Design review of the part built by this model. Coordinates are the model's own, in mm. A direction names the side the tool comes from. Coordinates: 2 decimals unless noted, no trailing zeros. Loops run counter-clockwise (first coordinate to the right, second up) from the corner with the lowest first, then second, coordinate; pieces in that order, holes last.
from build123d import *

# Parameters (mm, degrees)
F0_R     = 0.8
F1_DEPTH = 3
F2_R     = 0.8
F3_DEPTH = 30.501
F4_R     = 1


with BuildPart() as f1:
    # F0 (on Top) → F1 (new body)
    with BuildSketch(Plane.XY):
        with BuildLine():
            Line((13.5, 15.25), (-13.5, 15.25))
            ThreePointArc((-13.5, 15.25), (-14.56066, 14.81066), (-15, 13.75))
            Line((-15, 13.75), (-15, -13.75))
            ThreePointArc((-15, -13.75), (-14.56066, -14.81066), (-13.5, -15.25))
            Line((-13.5, -15.25), (13.5, -15.25))
            ThreePointArc((13.5, -15.25), (14.56066, -14.81066), (15, -13.75))
            Line((15, -13.75), (15, 13.75))
            ThreePointArc((15, 13.75), (14.56066, 14.81066), (13.5, 15.25))
        make_face()
        with Locations((-10, -10)):
            Circle(F0_R, mode=Mode.SUBTRACT)
        with Locations((10, -10)):
            Circle(F0_R, mode=Mode.SUBTRACT)
        with Locations((-10, 10)):
            Circle(F0_R, mode=Mode.SUBTRACT)
        with BuildLine():
            ThreePointArc((1.25, 9.921567), (7.5, 6.614378), (10, 0))
            ThreePointArc((10, 0), (7.5, -6.614378), (1.25, -9.921567))
            Line((1.25, -9.921567), (1.25, -10))
            ThreePointArc((1.25, -10), (0, -11.25), (-1.25, -10))
            Line((-1.25, -10), (-1.25, -9.921567))
            ThreePointArc((-1.25, -9.921567), (-10, 0), (-1.25, 9.921567))
            Line((-1.25, 9.921567), (-1.25, 10))
            ThreePointArc((-1.25, 10), (0, 11.25), (1.25, 10))
            Line((1.25, 10), (1.25, 9.921567))
        make_face(mode=Mode.SUBTRACT)
        with Locations((10, 10)):
            Circle(F0_R, mode=Mode.SUBTRACT)
    extrude(amount=F1_DEPTH)

    # F2 (on face) → F3 (cut, through all)
    with BuildSketch(Plane.XZ.offset(15.25)):
        with Locations((0, 1.5)):
            Circle(F2_R)
        with Locations((10, 1.5)):
            Circle(F2_R)
        with Locations((-10, 1.5)):
            Circle(F2_R)
    extrude(amount=-F3_DEPTH, mode=Mode.SUBTRACT)

    # F4
    f4_edges = [f1.edges().sort_by_distance(p)[0] for p in [
        (1.25, 9.921567, 1.5),
        (-1.25, 9.921567, 1.5),
        (-1.25, -9.921567, 1.5),
        (1.25, -9.921567, 1.5),
    ]]
    fillet(f4_edges, radius=F4_R)


solid = f1.part
Q1. Take a section at D-D, the plane z = 1.9. Give the number of separate pieces and of enclosed holes in the cut face, then the cut area to 3 significant figures.
Q2. For line 1 (Z direction, x = 10, y = -12); line 2 (X direction, y = 3, z = 1.5); line 3 (Y direction, x = -10.5, z = 0.65), list the stretches that pass through material, from the lowest coordinate up.
Q3. Clearance check with a flat-ended pin moving along its axis: pin 1 Ø1.8 at (x, y) = (-10, -10) entering from -Z. State where the tip first meets the part, or that it passes through.
Q4. Take a section at B-B, the plane y = -8.5. Write out the cut boundary in (x, z).
Q5. Take a section at A-A, the plane x = 0. Write out the cut boundary in (y, z), then the cut area to 3 significant figures.
Q6. Machinability: for faces 4 (the cylindrical face through (0.916, -10.85, 1.479)), 5 (the cylindrical face through (14.57, 14.8, 1.48)), which of the approach directions +Z, -Z, +X, -X, +Y, -Y give a long, thin tool a straight path to every point of the face, cutting with its end or side? Answer none if there is none.
Q7. The part is to be moulded in two halves that separate along X. For faces 1 (the flat face through (-15, 0, 1)), 2 (the cylindrical face through (-10.59, 10.54, 0.57)), 3 (the flat face through (-10.2, 0.2, 0)), say which applies: pulls with the +X half, pulls with the -X half, needs draft (parallel to the pull), parting line crosses it, or undercut.
Q8. Take a section at C-C, the plane y = -1. Write out the cut boundary in (x, z).
Entries:
1. separate pieces: 6
1. enclosed holes: 0
1. area: 504 mm2
2. line 1: z = 0 to 0.7, 2.3 to 3
2. line 2: x = -15 to -10.8, 10.8 to 15
2. line 3: y = -15.25 to -10.62, -9.38 to 9.38, 10.62 to 15.25
3. pin 1: stops at z = 0
4. outline: (-15, 0) - (-5.27, 0) - (-5.27, 3) - (-15, 3) - close; (5.27, 0) - (15, 0) - (15, 3) - (5.27, 3) - close; hole circle Ø1.6 at (-10, 1.5); hole circle Ø1.6 at (10, 1.5)
5. outline: (-15.25, 0) - (-11.25, 0) - (-11.25, 0.7) - (-15.25, 0.7) - close; (-15.25, 2.3) - (-11.25, 2.3) - (-11.25, 3) - (-15.25, 3) - close; (11.25, 0) - (15.25, 0) - (15.25, 0.7) - (11.25, 0.7) - close; (11.25, 2.3) - (15.25, 2.3) - (15.25, 3) - (11.25, 3) - close
5. area: 11.2 mm2
6. face 4: +Z, -Z
6. face 5: +Z, -Z, +X, +Y
7. face 1: pulls with the -X half
7. face 2: undercut
7. face 3: needs draft
8. outline: (-15, 0) - (-9.95, 0) - (-9.95, 0.7) arc R0.8 cw (long way) to (-9.95, 2.3) - (-9.95, 3) - (-15, 3) - close; (9.95, 0) - (15, 0) - (15, 3) - (9.95, 3) - (9.95, 2.3) arc R0.8 cw (long way) to (9.95, 0.7) - close
